```python
from build123d import *
from build123d.topology import SkipClean

# Parameters (mm, degrees)
EXTRUDE_1_DEPTH     = 2
SKETCH_2_R          = 1.1
CUT_EXTRUDE_1_DEPTH = 2
SKETCH_3_W          = 43.2
SKETCH_3_H          = 2
EXTRUDE_2_DEPTH     = 10
SKETCH_4_R          = 1
CUT_EXTRUDE_2_DEPTH = 2
SKETCH_5_R          = 3
SKETCH_5_R_2        = 1
EXTRUDE_3_DEPTH     = 2
CHAMFER_2_SIZE      = 1.6
CUT_EXTRUDE_3_DEPTH = 5.9
CUT_EXTRUDE_4_DEPTH = 5.9
SKETCH_9_R          = 1.2
CUT_EXTRUDE_5_DEPTH = 10
CUT_EXTRUDE_7_DEPTH = 10


with BuildPart() as part:
    # 草图1 → 凸台-拉伸1 (new body)
    with BuildSketch(Plane(origin=(0, 0, 0), x_dir=(1, 0, 0), z_dir=(0, 1, 0))):
        Polygon((24.1, -12.5), (27.5, -8), (27.5, -2.885), (26.2, -1.65), (26.2, 1.65), (27.5, 2.885), (27.5, 8), (24.1, 12.5), (21.6, 12.5), (21.6, 15.18), (-21.6, 15.18), (-21.6, 12.5), (-24.1, 12.5), (-27.5, 8), (-27.5, 2.885), (-26.2, 1.65), (-26.2, -1.65), (-27.5, -2.885), (-27.5, -8), (-24.1, -12.5), (-21.6, -12.5), (-21.6, -15.18), (21.6, -15.18), (21.6, -12.5), align=None)
        Polygon((17.05, -9.2), (6.84, -9.2), (3.5, -6.2), (-3.5, -6.2), (-6.84, -9.2), (-17.05, -9.2), (-21.75, -4.5), (-21.75, 4.5), (-17.05, 9.2), (-6.84, 9.2), (-3.5, 6.2), (3.5, 6.2), (6.84, 9.2), (17.05, 9.2), (21.75, 4.5), (21.75, -4.5), align=None, mode=Mode.SUBTRACT)
    extrude(amount=EXTRUDE_1_DEPTH)

    # 草图2 → 切除-拉伸1 (cut)
    with BuildSketch(Plane(origin=(0, 2, 0), x_dir=(1, 0, 0), z_dir=(0, 1, 0))):
        with Locations(Location((20.742981447, -8.464435144, 0), (0, 0, 270))):
            Circle(SKETCH_2_R)
        with Locations(Location((-20.742981447, 8.464435144, 0), (0, 0, 270))):
            Circle(SKETCH_2_R)
        with BuildLine():
            Line((21.75, 8.021813823), (21.75, 8.907056465))
            ThreePointArc((21.75, 8.907056465), (21.667117231, 9.061069917), (21.560871624, 9.2))
            Line((21.560871624, 9.2), (21.354867257, 9.2))
            Line((21.354867257, 9.2), (21.446447919, 9.310091648))
            ThreePointArc((21.446447919, 9.310091648), (19.672301899, 8.21215493), (21.75, 8.021813823))
        make_face()
        with Locations(Location((-20.742981447, -8.464435144, 0), (0, 0, 270))):
            Circle(SKETCH_2_R)
    extrude(amount=-CUT_EXTRUDE_1_DEPTH, mode=Mode.SUBTRACT)

    # 草图3 → 凸台-拉伸2 (add)
    with BuildSketch(Plane.XZ):
        with Locations((0, -14.18)):
            Rectangle(SKETCH_3_W, SKETCH_3_H)
        with Locations((0, 14.18)):
            Rectangle(SKETCH_3_W, SKETCH_3_H)
    extrude(amount=EXTRUDE_2_DEPTH)

    # 草图4 → 切除-拉伸2 (cut)
    with BuildSketch(Plane(origin=(0, 0, -15.18), x_dir=(-1, 0, 0), z_dir=(0, 0, -1))):
        with Locations((-17.45, -5.85)):
            Circle(SKETCH_4_R)
        with BuildLine():
            ThreePointArc((-17.45, -10), (-20.384493142, -8.784493142), (-21.6, -5.85))
            Line((-21.6, -5.85), (-21.6, -10))
            Line((-21.6, -10), (-17.45, -10))
        make_face()
        with Locations((17.45, -5.85)):
            Circle(SKETCH_4_R)
        with BuildLine():
            Line((21.6, -10), (21.6, -5.85))
            ThreePointArc((21.6, -5.85), (20.384493142, -8.784493142), (17.45, -10))
            Line((17.45, -10), (21.6, -10))
        make_face()
    extrude(amount=-CUT_EXTRUDE_2_DEPTH, mode=Mode.SUBTRACT)

    # 草图5 → 凸台-拉伸3 (add)
    # profile 1 of 2: a face of its own
    with BuildSketch(Plane.XY.offset(-13.18)):
        with Locations(Location((17.45, -5.85, 0), (0, 0, 180))):
            Circle(SKETCH_5_R)
        with Locations(Location((17.45, -5.85, 0), (0, 0, 180))):
            Circle(SKETCH_5_R_2, mode=Mode.SUBTRACT)
    # profile 2 of 2: a face of its own
    with BuildSketch(Plane.XY.offset(-13.18)):
        with Locations(Location((-17.45, -5.85, 0), (0, 0, 180))):
            Circle(SKETCH_5_R)
        with Locations(Location((-17.45, -5.85, 0), (0, 0, 180))):
            Circle(SKETCH_5_R_2, mode=Mode.SUBTRACT)
    extrude(amount=EXTRUDE_3_DEPTH)

    # 倒角2
    chamfer_2_edges = [part.edges().sort_by_distance(p)[0] for p in [
        (0, 2, 15.18),
        (0, 0, 13.18),
        (0, 0, -13.18),
        (0, 2, -15.18),
    ]]
    chamfer(chamfer_2_edges, length=CHAMFER_2_SIZE)

    # 草图7 → 切除-拉伸3 (cut)
    with BuildSketch(Plane(origin=(21.6, 0, 0), x_dir=(0, 0, -1), z_dir=(1, 0, 0))):
        Polygon((-12.5, -0.92), (-11.58, 0), (-12.5, 0), align=None)
        Polygon((12.5, 0), (11.58, 0), (12.5, -0.92), align=None)
    extrude(amount=CUT_EXTRUDE_3_DEPTH, mode=Mode.SUBTRACT)

    # 草图8 → 切除-拉伸4 (cut)
    with BuildSketch(Plane.ZY.offset(27.5)):
        Polygon((12.5, 0), (11.58, 0), (12.5, -0.92), align=None)
        Polygon((-12.5, -0.92), (-11.58, 0), (-12.5, 0), align=None)
    extrude(amount=-CUT_EXTRUDE_4_DEPTH, mode=Mode.SUBTRACT)

    # 草图9 → 切除-拉伸5 (cut)
    with BuildSketch(Plane.XY.offset(15.18)):
        with Locations((-16.15, -5.8)):
            Circle(SKETCH_9_R)
        with Locations((16.15, -5.8)):
            Circle(SKETCH_9_R)
    extrude(amount=-CUT_EXTRUDE_5_DEPTH, mode=Mode.SUBTRACT)

    # 草图11 → 切除-拉伸7 (cut)
    with SkipClean():  # the faces are left unmerged after this step: merging them gives an invalid solid
        with BuildSketch(Plane(origin=(0, 2, 0), x_dir=(1, 0, 0), z_dir=(0, 1, 0))):
            with BuildLine():
                Line((21.446447919, 9.310091648), (21.354867257, 9.2))
                Line((21.354867257, 9.2), (21.560871624, 9.2))
                ThreePointArc((21.560871624, 9.2), (21.667117231, 9.061069917), (21.75, 8.907056465))
                Line((21.75, 8.907056465), (21.75, 8.021813823))
                ThreePointArc((21.75, 8.021813823), (19.672301899, 8.21215493), (21.446447919, 9.310091648))
            make_face()
            with BuildLine():
                Line((21.75, 8.907056465), (21.75, 8.021813823))
                ThreePointArc((21.75, 8.021813823), (21.819485141, 8.238294047), (21.842981447, 8.464435144))
                ThreePointArc((21.842981447, 8.464435144), (21.819485141, 8.690576241), (21.75, 8.907056465))
            make_face()
            with BuildLine():
                ThreePointArc((21.560871624, 9.2), (21.505648843, 9.257113164), (21.446447919, 9.310091648))
                Line((21.446447919, 9.310091648), (21.354867257, 9.2))
                Line((21.354867257, 9.2), (21.560871624, 9.2))
            make_face()
        extrude(amount=-CUT_EXTRUDE_7_DEPTH, mode=Mode.SUBTRACT)


solid = part.part
```
Design review of the part built by this model. Coordinates are the model's own, in mm. A direction names the side the tool comes from. Give positions to 0.01 mm unless a question says otherwise; leave off trailing zeros. Order: outer loops, then holes, each group sorted by start corner. A loop starts at its lowest first (then second) coordinate and runs counter-clockwise, first axis right, second up. Notation, with made-up numbers: (67, 4) - (71, 4) arc R27 cw to (71, 23) - close; hole circle Ø9 at (25.25, 67). An arc over 180 degrees is marked (long way). Use a Markdown table: item, result. Add a question column.
(1) Add section C-C on x = -11.5. Give the boundary of the cut face in (y, z), then the cut area to 3 significant figures.
(2) Mouldability with a two-part tool opening along Y and no side actions: class faces 4 (the face through (-17, -7, -11.18)), 5 (the face through (-17.35, -5.75, 14.19)), 6 (the face through (20.35, -8.82, -14.19)) as +Y half, -Y half, draft (parallel to the pull), parting line (faces both ways), or undercut.
(3) Add section A-A on x = -2. Give the boundary of the cut face in (y, z).
(4) Add section B-B on z = -5.5. Give the boundary of the cut face in (x, y), then the cut area to 3 significant figures.
(5) Clearance check with flat-ended pins moving along their axes: P1, Ø1.6, axis at x = -22.5, y = 1, coming from the +Z side; P2, Ø10, axis at x = 4, z = 4.5, coming from the -Y side; P3, Ø0.7, axis at y = -0.5, z = 12, coming from the -X side. State where each tip first meets the part, or that it passes through.
(6) Wall thickness on probe 1 along Z at (x, y) = (-17, -8); probe 2 along Z at (x, y) = (3, -6.5); probe 3 along Y at (x, z) = (17.45, -12.25): over which ranges is each line inside the solid? List them lowest first. Write a range as [from, to].
(7) Machinability: for faces 1 (the face through (0, -6, 13.18)), 2 (the face through (23, 1, 12.5)), 3 (the face through (-21.75, 1, 0)), which of the approach directions +Z, -Z, +X, -X, +Y, -Y give a long, thin tool a straight path to every point of the face, cutting with its end or side? Answer none if there is none.
Report:
| question | item | result |
|---|---|---|
| 1 | outline | (-10, -15.18) - (0.4, -15.18) - (2, -13.58) - (2, -9.2) - (0, -9.2) - (0, -11.58) - (-1.6, -13.18) - (-10, -13.18) - close; (-10, 13.18) - (-1.6, 13.18) - (0, 11.58) - (0, 9.2) - (2, 9.2) - (2, 13.58) - (0.4, 15.18) - (-10, 15.18) - close |
| 1 | area | 63.9 mm² |
| 2 | face 4 | draft |
| 2 | face 5 | undercut |
| 2 | face 6 | -Y half |
| 3 | outline | (-10, -15.18) - (0.4, -15.18) - (2, -13.58) - (2, -6.2) - (0, -6.2) - (0, -11.58) - (-1.6, -13.18) - (-10, -13.18) - close; (-10, 13.18) - (-1.6, 13.18) - (0, 11.58) - (0, 6.2) - (2, 6.2) - (2, 13.58) - (0.4, 15.18) - (-10, 15.18) - close |
| 4 | outline | (-27.5, 0) - (-20.75, 0) - (-20.75, 2) - (-27.5, 2) - close; (20.75, 0) - (27.5, 0) - (27.5, 2) - (20.75, 2) - close |
| 4 | area | 27.0 mm² |
| 5 | P1 | stops at z = 12.5 |
| 5 | P2 | stops at y = 0 |
| 5 | P3 | stops at x = -21.6 |
| 6 | probe 1 | z = [-15.18, -11.18], [13.18, 15.18] |
| 6 | probe 2 | z = [-15.18, -13.18], [13.18, 15.18] |
| 6 | probe 3 | y = [-8.85, -6.85], [-4.85, -2.85], [-0.67, 2] |
| 7 | face 1 | +X, -X, -Y |
| 7 | face 2 | +Z, +X, +Y, -Y |
| 7 | face 3 | +Y, -Y |
